```python
from build123d import *

# Parameters (mm, degrees)
SKETCH_W        = 25
SKETCH_H        = 32
SKETCH_R        = 0.75
SKETCH_R_2      = 0.5
PAD_DEPTH       = 4
SKETCH001_W     = 5
SKETCH001_H     = 32
POCKET_DEPTH    = 1
SKETCH002_W     = 11
SKETCH002_H     = 20.5
POCKET001_DEPTH = 2
SKETCH003_W     = 1
SKETCH003_H     = 12
POCKET002_DEPTH = 1


with BuildPart() as part:
    # Sketch → Pad (new body)
    with BuildSketch(Plane.XY):
        Rectangle(SKETCH_W, SKETCH_H)
        with Locations((-10, 13)):
            Circle(SKETCH_R, mode=Mode.SUBTRACT)
        with Locations((-10, -13)):
            Circle(SKETCH_R, mode=Mode.SUBTRACT)
        with Locations((2.34, 4.5)):
            Circle(SKETCH_R_2, mode=Mode.SUBTRACT)
        with Locations((4.88, 4.5)):
            Circle(SKETCH_R_2, mode=Mode.SUBTRACT)
        with Locations((7.42, 4.5)):
            Circle(SKETCH_R_2, mode=Mode.SUBTRACT)
        with Locations((9.96, 4.5)):
            Circle(SKETCH_R_2, mode=Mode.SUBTRACT)
    extrude(amount=PAD_DEPTH)

    # Sketch001 (on Face11 of Pad) → Pocket (cut)
    with BuildSketch(Plane(origin=(0, 0, 0), x_dir=(1, 0, 0), z_dir=(0, 0, -1))):
        with Locations((-10, 0)):
            Rectangle(SKETCH001_W, SKETCH001_H)
    extrude(amount=-POCKET_DEPTH, mode=Mode.SUBTRACT)

    # Sketch002 (on Face6 of Pocket) → Pocket001 (cut)
    with BuildSketch(Plane.XY.offset(4)):
        with Locations((6, -4.25)):
            Rectangle(SKETCH002_W, SKETCH002_H)
    extrude(amount=-POCKET001_DEPTH, mode=Mode.SUBTRACT)

    # Sketch003 (on Face4 of Pocket001) → Pocket002 (cut)
    with BuildSketch(Plane(origin=(0, 0, 0), x_dir=(1, 0, 0), z_dir=(0, 0, -1))):
        with Locations((2.33, -10)):
            Rectangle(SKETCH003_W, SKETCH003_H)
        with Locations((4.87, -10)):
            Rectangle(SKETCH003_W, SKETCH003_H)
        with Locations((7.41, -10)):
            Rectangle(SKETCH003_W, SKETCH003_H)
        with Locations((9.95, -10)):
            Rectangle(SKETCH003_W, SKETCH003_H)
    extrude(amount=-POCKET002_DEPTH, mode=Mode.SUBTRACT)


solid = part.part
```
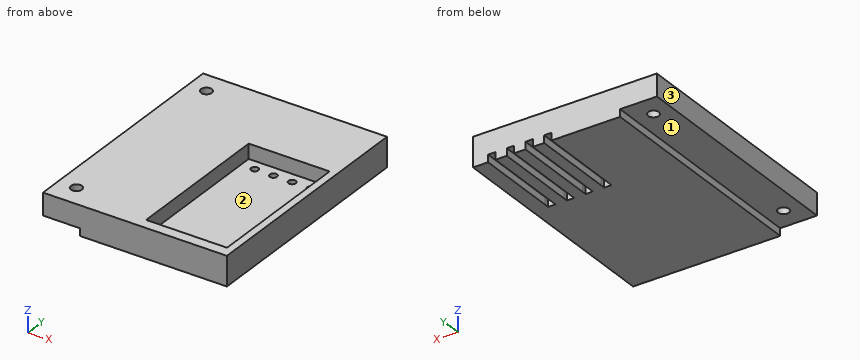
Part model, mm, in its own coordinate system. Face numbers are marked on the shaded views. Give positions to 0.01 mm unless a question says otherwise; leave off trailing zeros. Loops run counter-clockwise (first coordinate to the right, second up) from the corner with the lowest first, then second, coordinate; pieces in that order, holes last. Notation, with made-up numbers: M 20.25,44 L 65.25,44 A21 ccw 65.25,63 Z; hole C -2,58 d3. An arc over 180 degrees is marked long. Return JSON: item names as keys, results as strings.
1) Flat gauge pins, fed straight in: pin 1 Ø4 at (x, y) = (7.5, 10) entering from -Z; pin 2 Ø0.5 at (x, y) = (10, 8) entering from -Z. Where does each tip first touch, or does it go through?
Calculated:
{"pin 1": "stops at z = 0", "pin 2": "stops at z = 1"}
2) Saw through at C-C, the plane z = 2.8. List the corners of the cut face in (x, y), then the cut area to 3 significant figures.
Calculated:
{"outline": "M -12.5,-16 L 12.5,-16 L 12.5,16 L -12.5,16 Z; hole C -10,-13 d1.5; hole C -10,13 d1.5; hole M 0.5,-14.5 L 11.5,-14.5 L 11.5,6 L 0.5,6 Z", "area": "571 mm2"}
3) Saw through at D-D, the plane x = 8.75. List the corners of the cut face in (y, z).
Calculated:
{"outline": "M -16,0 L 16,0 L 16,4 L 6,4 L 6,2 L -14.5,2 L -14.5,4 L -16,4 Z"}
4) Pull direction X, two halves, no side cores. Call the marked faces 1, 2 and 3: released by +X, released by -X, zero draft, split by the parting line, or undercut.
Calculated:
{"face 1": "zero draft", "face 2": "undercut", "face 3": "released by -X"}
5) Drill centre lines: line 1 (X direction, y = 4.5, z = 0.4); line 2 (Y direction, x = -10, z = 1.95); line 3 (X direction, y = 4.5, z = 1.25). Where is each one in solid material? Low to high.
Calculated:
{"line 1": "x = -7.5 to 1.83, 2.84 to 4.37, 5.38 to 6.91, 7.92 to 9.45, 10.46 to 12.5", "line 2": "y = -16 to -13.75, -12.25 to 12.25, 13.75 to 16", "line 3": "x = -12.5 to 1.84, 2.84 to 4.38, 5.38 to 6.92, 7.92 to 9.46, 10.46 to 12.5"}
6) Saw through at B-B, the plane x = -10. List the corners of the cut face in (y, z), then the cut area to 3 significant figures.
Calculated:
{"outline": "M -16,1 L -13.75,1 L -13.75,4 L -16,4 Z; M -12.25,1 L 12.25,1 L 12.25,4 L -12.25,4 Z; M 13.75,1 L 16,1 L 16,4 L 13.75,4 Z", "area": "87.0 mm2"}
7) Saw through at A-A, the plane y = -13. List the corners of the cut face in (x, z), then the cut area to 3 significant figures.
Calculated:
{"outline": "M -12.5,1 L -10.75,1 L -10.75,4 L -12.5,4 Z; M -9.25,1 L -7.5,1 L -7.5,0 L 12.5,0 L 12.5,4 L 11.5,4 L 11.5,2 L 0.5,2 L 0.5,4 L -9.25,4 Z", "area": "68.5 mm2"}
